```python
from build123d import *

# Parameters (mm, degrees)
ESQUISSE1_R                  = 3
BOSS_EXTRU_1_DEPTH           = 13
ESQUISSE2_R                  = 1
ENL_V_MAT_EXTRU_1_DEPTH      = 14.674794331
ENL_V_MAT_EXTRU_3_DEPTH      = 14.674794331
ENL_V_MAT_EXTRU_3_DEPTH_BACK = 14.674794331
ESQUISSE4_R                  = 1.25


with BuildPart() as part:
    # Esquisse1 → Boss.-Extru.1 (new body)
    with BuildSketch(Plane(origin=(0, 0, 0), x_dir=(1, 0, 0), z_dir=(0, 1, 0))):
        with Locations(Location((0, 0, 0), (0, 0, 270))):
            Circle(ESQUISSE1_R)
    extrude(amount=BOSS_EXTRU_1_DEPTH)

    # Esquisse2 → Enlèv. mat.-Extru.1 (cut, through all)
    with BuildSketch(Plane.XZ):
        with Locations(Location((0, 0, 0), (0, 0, 270))):
            Circle(ESQUISSE2_R)
    extrude(amount=-ENL_V_MAT_EXTRU_1_DEPTH, mode=Mode.SUBTRACT)

    # Esquisse4 → Enlèv. mat.-Extru.3 (cut, two sides: drawn at the far end of the back side and taken through both)
    with BuildSketch(Plane(origin=(0, 0, 0), x_dir=(0, 0, -1), z_dir=(1, 0, 0)).offset(-ENL_V_MAT_EXTRU_3_DEPTH_BACK)):
        with Locations((0, 4)):
            Circle(ESQUISSE4_R)
    extrude(amount=ENL_V_MAT_EXTRU_3_DEPTH + ENL_V_MAT_EXTRU_3_DEPTH_BACK, mode=Mode.SUBTRACT)


solid = part.part
```
Work out the finished part from the listing and answer in its coordinate system (mm). Give positions to 0.01 mm unless a question says otherwise; leave off trailing zeros. Loops run counter-clockwise (first coordinate to the right, second up) from the corner with the lowest first, then second, coordinate; pieces in that order, holes last. Notation, with made-up numbers: (-13, -40) -> (-3, -40) arc R29 cw to (-3, -20) -> close; hole circle Ø11 at (-20, 7.25). An arc over 180 degrees is marked (long way). Write item = value, one per line. Start each with the question number.
(1) Find section C-C on y = 7.5. Give the vertices of the cut face in (x, z).
(2) Find section B-B on x = 0. Give the vertices of the cut face in (y, z).
(3) Find the intervals of material crossed by probe 1 along X at (y, z) = (9.5, 0); probe 2 along Y at (x, z) = (-1, 1); probe 3 along X at (y, z) = (5.5, -0.5), in increasing order. Write a range as from..to.
(4) Given pin 1 Ø1.2 at (x, z) = (0, 0) entering from +Y, flat-ended and moving along its own axis, determine where the tip first touches the part or whether it passes through.
(5) Find section D-D on x = -1.5. Give the vertices of the cut face in (y, z).
(6) The mould has two halves that part along Y. Classify faces 1 (the cylindrical face through (0, 2, -1)), 2 (the cylindrical face through (-0.04, 4.05, 1.25)), 3 (the flat face through (1, 0, -1)): +Y half, -Y half, draft (parallel to the pull), parting line (faces both ways), or undercut.
(7) Find section A-A on z = 0. Give the vertices of the cut face in (x, y), and give its area (3 significant figures).
From the geometry:
q1.outline = circle Ø6 at (0, 0); hole circle Ø2 at (0, 0)
q2.outline = (0, -3) -> (13, -3) -> (13, -1) -> (4.75, -1) arc R1.25 cw to (3.25, -1) -> (0, -1) -> close; (0, 1) -> (3.25, 1) arc R1.25 cw to (4.75, 1) -> (13, 1) -> (13, 3) -> (0, 3) -> close
q3.probe_1 = -3..-1, 1..3
q3.probe_2 = 0..3.25, 4.75..13
q3.probe_3 = -2.96..-0.87, 0.87..2.96
q4.pin_1 = through
q5.outline = (0, -2.6) -> (13, -2.6) -> (13, 2.6) -> (0, 2.6) -> close; hole circle Ø2.5 at (4, 0)
q6.face_1 = draft
q6.face_2 = undercut
q6.face_3 = -Y half
q7.outline = (-3, 0) -> (-1, 0) -> (-1, 2.75) -> (-3, 2.75) -> close; (-3, 5.25) -> (-1, 5.25) -> (-1, 13) -> (-3, 13) -> close; (1, 0) -> (3, 0) -> (3, 2.75) -> (1, 2.75) -> close; (1, 5.25) -> (3, 5.25) -> (3, 13) -> (1, 13) -> close
q7.area = 42.0 mm^2
